Can you work these out from the drawing? Everything is in mm from the part's minimum corner. A direction names the side the tool comes from. Round coordinates to 2 decimals unless told otherwise and drop trailing zeros. Write each loop counter-clockwise with the first axis right and the second up, starting at its lowest first coordinate (ties: lowest second). Pieces come first, ordered by that corner, then holes. Notation, with made-up numbers: M 86,71.25 L 110,71.25 A19 ccw 110,76.25 Z; hole C 66,-21 d10. An arc over 180 degrees is marked long. Use one line per item in the form item = value. Start each with the question number.
Q1. I'm going to push flat-ended pins straight in: pin 1 Ø7.5 at (y, z) = (51, 39) entering from -X; pin 2 Ø11 at (x, z) = (47, 20.5) entering from -Y; pin 3 Ø9.5 at (y, z) = (27.5, 38.5) entering from +X. Where does each tip first touch, or does it pass through?
Q2. I need wall thicknesses on line 1 along X through (y, z) = (36, 46.5); line 2 along Z through (x, y) = (24.5, 27); line 3 along Y through (x, z) = (47.5, 56). Which ranges of each line are inside material? Lowest first, please. Write a range as from..to.
Q3. I want a section at D-D on y = 8. List the corners of the cut face in (x, z) for me.
Q4. I want a section at B-B on x = 45. List the corners of the cut face in (y, z) for me, and give its area (3 significant figures).
Q5. I want a section at C-C on x = 23. List the corners of the cut face in (y, z) for me, and give its area (3 significant figures).
Q6. I want a section at A-A on z = 35. List the corners of the cut face in (x, y) for me.
Q7. For the marked faces 1, 2, 3, 4 and 5, which set-ups out of +Z, -Z, +X, -X, +Y, -Y let a thin tool reach every point of the face, with its end or its side?
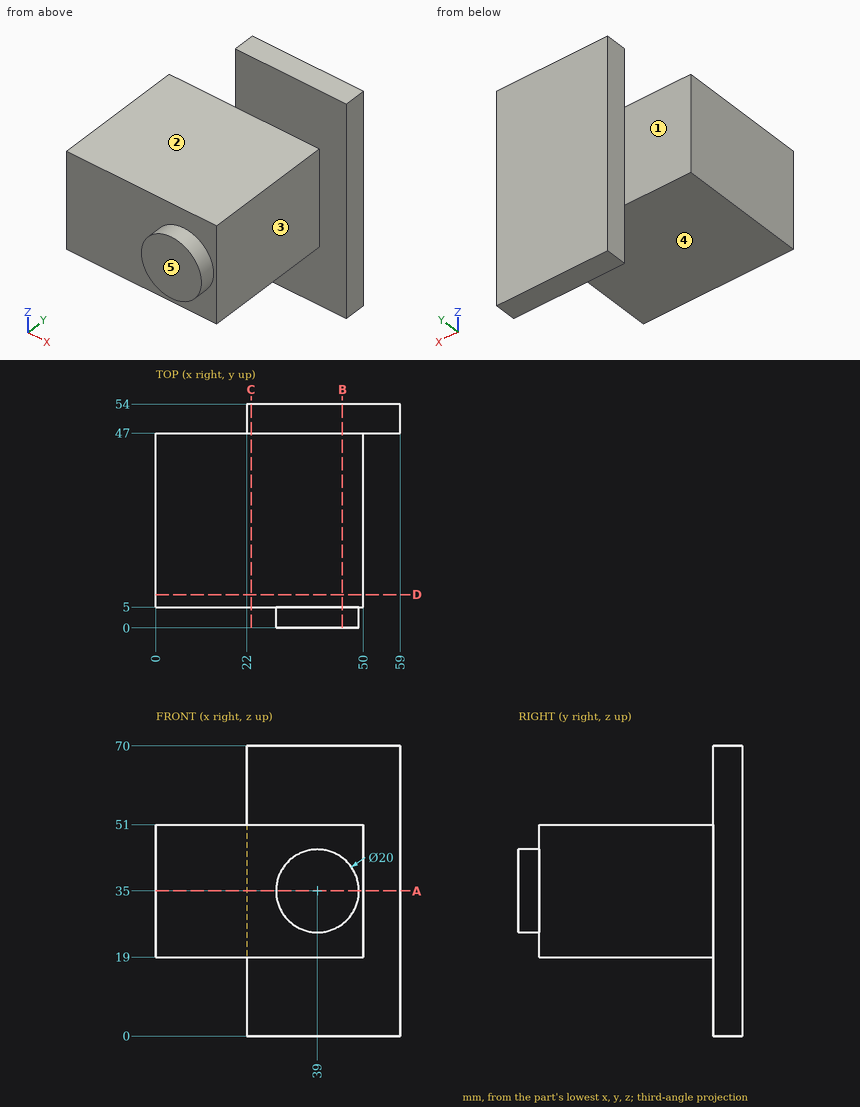
Reported:
q1.pin_1 = 22
q1.pin_2 = 5
q1.pin_3 = 50
q2.line_1 = 0..50
q2.line_2 = 19..51
q2.line_3 = 47..54
q3.outline = M 0,19 L 50,19 L 50,51 L 0,51 Z
q4.outline = M 0,27 L 5,27 L 5,19 L 47,19 L 47,0 L 54,0 L 54,70 L 47,70 L 47,51 L 5,51 L 5,43 L 0,43 Z
q4.area = 1,910 mm^2
q5.outline = M 5,19 L 47,19 L 47,0 L 54,0 L 54,70 L 47,70 L 47,51 L 5,51 Z
q5.area = 1,830 mm^2
q6.outline = M 0,5 L 29,5 L 29,0 L 49,0 L 49,5 L 50,5 L 50,47 L 59,47 L 59,54 L 22,54 L 22,47 L 0,47 Z
q7.face_1 = +Z, -Z, -X, +Y
q7.face_2 = +Z, +X, -X, -Y
q7.face_3 = +Z, -Z, +X, -Y
q7.face_4 = -Z, +X, -X, -Y
q7.face_5 = +Z, -Z, +X, -X, -Y
